Job drawing, mm, ordinate dimensions from the low corner. One solid piece. Coordinates: 2 decimals unless noted, no trailing zeros. Loops run counter-clockwise (first coordinate to the right, second up) from the corner with the lowest first, then second, coordinate; pieces in that order, holes last. Notation, with made-up numbers: (59.25, 0.25) -> (84.25, 0.25) arc R21 ccw to (84.25, 21.25) -> close; hole circle Ø10 at (47.5, 68). An arc over 180 degrees is marked (long way). Answer as CSV lines item,"result". Start each with the question number.
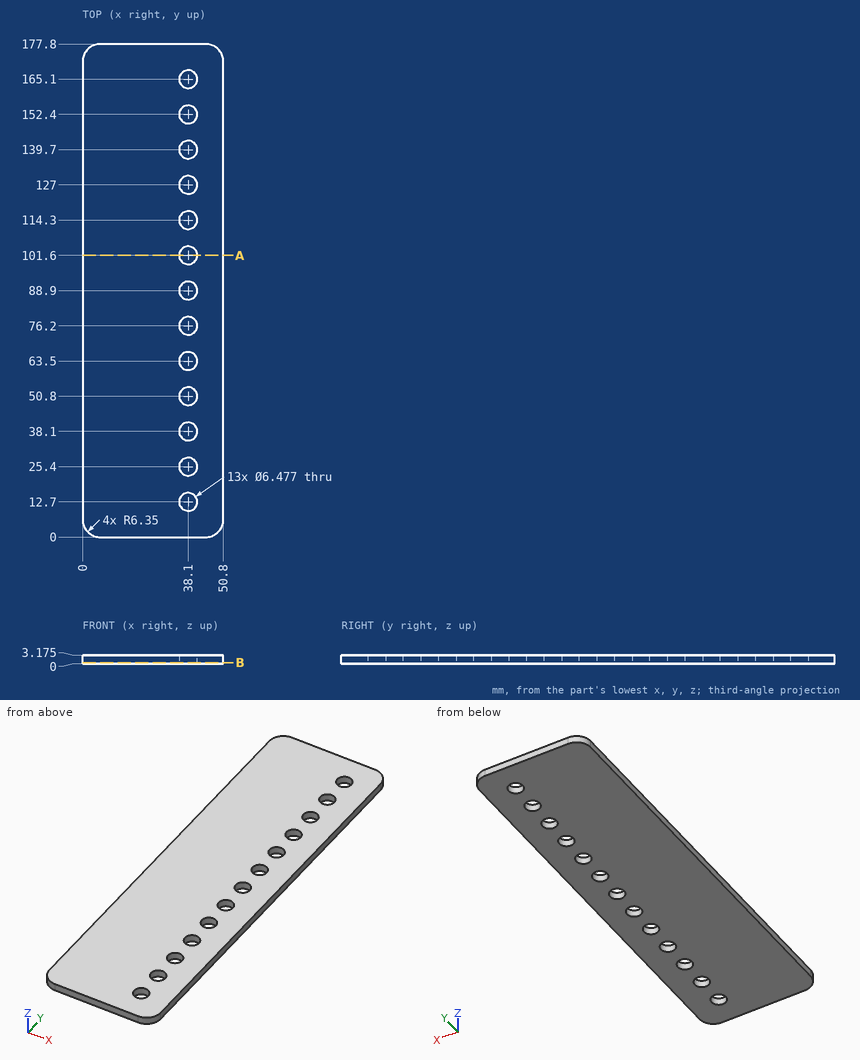
Item 1: Saw through at A-A (y = 101.6). Write the cut outline in (x, z) (1 decimal), plus the area to 3 significant figures.
Item 2: Wall check: probe 1 along X at (y, z) = (114, 0.5); probe 2 along Y at (x, z) = (6, 0.55); probe 3 along X at (y, z) = (117, 1.4). Give the ranges that are in metal, low to high.
Item 3: Saw through at B-B (z = 0.5). Count the separate pieces of the cut face and the enclosed holes in it, plus the area to 3 significant figures.
Geometry check:
1,outline,"(0, 0) -> (34.9, 0) -> (34.9, 3.2) -> (0, 3.2) -> close; (41.3, 0) -> (50.8, 0) -> (50.8, 3.2) -> (41.3, 3.2) -> close"
1,area,"141 mm2"
2,probe 1,"0 to 34.88, 41.32 to 50.8"
2,probe 2,"0.01 to 177.79"
2,probe 3,"0 to 36.31, 39.89 to 50.8"
3,separate pieces,"1"
3,enclosed holes,"13"
3,area,"8,570 mm2"
